```python
from build123d import *

# Parameters (mm, degrees)
SALIENTE_EXTRUIR1_DEPTH = 6
CROQUIS3_R              = 1.25
CORTAR_EXTRUIR1_DEPTH   = 4
CROQUIS4_R              = 1.25
CORTAR_EXTRUIR2_DEPTH   = 4
CROQUIS5_R              = 1.6
CORTAR_EXTRUIR3_DEPTH   = 6


with BuildPart() as part:
    # Croquis1 → Saliente-Extruir1 (new body)
    with BuildSketch(Plane.XY):
        Polygon((0, 0), (0, 20), (4, 20), (4, 12), (12, 4), (20, 4), (20, 0), align=None)
    extrude(amount=SALIENTE_EXTRUIR1_DEPTH)

    # Croquis3 → Cortar-Extruir1 (cut)
    with BuildSketch(Plane(origin=(0, 4, 0), x_dir=(1, 0, 0), z_dir=(0, 1, 0))):
        with Locations(Location((16, -3, 0), (0, 0, 180))):
            Circle(CROQUIS3_R)
    extrude(amount=-CORTAR_EXTRUIR1_DEPTH, mode=Mode.SUBTRACT)

    # Croquis4 → Cortar-Extruir2 (cut)
    with BuildSketch(Plane(origin=(4, 0, 0), x_dir=(0, 0, -1), z_dir=(1, 0, 0))):
        with Locations(Location((-3, 16, 0), (0, 0, 90))):
            Circle(CROQUIS4_R)
    extrude(amount=-CORTAR_EXTRUIR2_DEPTH, mode=Mode.SUBTRACT)

    # Croquis5 → Cortar-Extruir3 (cut)
    with BuildSketch(Plane.XY.offset(6)):
        with Locations((16, 5)):
            Circle(CROQUIS5_R)
        with Locations((5, 16)):
            Circle(CROQUIS5_R)
    extrude(amount=-CORTAR_EXTRUIR3_DEPTH, mode=Mode.SUBTRACT)


solid = part.part
```
The model under review builds one solid part; all positions refer to its coordinate system, in mm. A direction names the side the tool comes from. Coordinates: 2 decimals unless noted, no trailing zeros. Write each loop counter-clockwise with the first axis right and the second up, starting at its lowest first coordinate (ties: lowest second). Pieces come first, ordered by that corner, then holes. Notation, with made-up numbers: (36.5, -0.75) - (70.5, -0.75) arc R13 ccw to (70.5, 10.25) - close; hole circle Ø2 at (-13, 41). An arc over 180 degrees is marked (long way). Answer in a Markdown table with one row per item. Add a question column.
Q1. Consider section D-D on y = 2.75. Give the boundary of the cut face in (x, z).
Q2. Draft analysis for pull direction Z (two halves, no side actions). For faces 1 (the face through (14.845, 2.028, 2.521)), 2 (the face through (10, 0, 3)), 3 (the face through (6, 8, 0)), 4 (the face through (6, 8, 6)), state which applies: +Z half, -Z half, draft (parallel to the pull), parting line (faces both ways), or undercut.
Q3. For faces 5 (the face through (19, 4, 3)), 6 (the face through (3.4, 16, 4.9)), list the 3-axis set-ups (+Z, -Z, +X, -X, +Y, -Y) from which the entire face can be reached by the end or side of a thin tool; tool diameter is ignored.
Q4. Consider section A-A on x = 16. Give the boundary of the cut face in (y, z), then the cut area to 3 significant figures.
Q5. Clearance check with flat-ended pins moving along their axes: pin 1 (2 mm diameter, centred on x = 14, z = 4, fed in from +Y); pin 2 (0.8 mm diameter, centred on y = 19, z = 3, fed in from +X); pin 3 (2 mm diameter, centred on x = 11.5, z = 3, fed in from +Y). State where each tip first meets the part, or that it passes through.
Q6. Consider section C-C on z = 2. Give the boundary of the cut face in (x, y), then the cut area to 3 significant figures.
Q7. To check wall thickness, follow line 1 along X through (y, z) = (1.55, 3); line 2 along Z through (x, y) = (16, 2.35). State the ranges of each line that lie inside material, in increasing order. Write a range as from..to.
Answers below:
| question | item | result |
|---|---|---|
| 1 | outline | (0, 0) - (20, 0) - (20, 6) - (0, 6) - close; hole circle Ø2.5 at (16, 3) |
| 2 | face 1 | undercut |
| 2 | face 2 | draft |
| 2 | face 3 | -Z half |
| 2 | face 4 | +Z half |
| 3 | face 5 | +Z, -Z, +X, +Y |
| 3 | face 6 | +Z, -Z, +X |
| 4 | outline | (0, 0) - (3.4, 0) - (3.4, 1.75) - (0, 1.75) - close; (0, 4.25) - (3.4, 4.25) - (3.4, 6) - (0, 6) - close |
| 4 | area | 11.9 mm² |
| 5 | pin 1 | y = 4 |
| 5 | pin 2 | x = 4 |
| 5 | pin 3 | y = 5.5 |
| 6 | outline | (0, 0) - (15.25, 0) - (15.25, 3.59) arc R1.6 cw to (14.75, 4) - (12, 4) - (4, 12) - (4, 14.75) arc R1.6 cw to (3.59, 15.25) - (0, 15.25) - close; (0, 16.75) - (3.59, 16.75) arc R1.6 cw to (4, 17.25) - (4, 20) - (0, 20) - close; (16.75, 0) - (20, 0) - (20, 4) - (17.25, 4) arc R1.6 cw to (16.75, 3.59) - close |
| 6 | area | 164 mm² |
| 7 | line 1 | 0..14.75, 17.25..20 |
| 7 | line 2 | 0..1.75, 4.25..6 |
